Verification items for the finished model (mm, model axes). A direction names the side the tool comes from. Coordinates: 2 decimals unless noted, no trailing zeros. Order: outer loops, then holes, each group sorted by start corner. A loop starts at its lowest first (then second) coordinate and runs counter-clockwise, first axis right, second up. Notation, with made-up numbers: (-17, -5.75) - (11, -5.75) arc R13 cw to (11, 4.25) - close; hole circle Ø5 at (26, 62.5). An arc over 180 degrees is marked (long way). One line per question, with ' | ' between items. Start each with the question number.
from build123d import *

# Parameters (mm, degrees)
RESSALTO_EXTRUS_O1_DEPTH = 2
CORTE_EXTRUS_O1_DEPTH    = 0.1
ESBO_O3_W                = 8
ESBO_O3_H                = 18
ESBO_O3_W_2              = 6.2
ESBO_O3_H_2              = 8.2
RESSALTO_EXTRUS_O2_DEPTH = 1
ESBO_O4_W                = 3.2
ESBO_O4_H                = 1
RESSALTO_EXTRUS_O3_DEPTH = 1.8
ESBO_O5_W                = 3.2
ESBO_O5_H                = 1.4
RESSALTO_EXTRUS_O4_DEPTH = 3
CHANFRO1_SIZE            = 2
CHANFRO1_SIZE2           = 0.388760618
FILETE1_R                = 0.4
ESBO_O6_W                = 3
ESBO_O6_H                = 0.8
RESSALTO_EXTRUS_O5_DEPTH = 1.4
ESBO_O7_W                = 3.5
ESBO_O7_H                = 1.2
CORTE_EXTRUS_O2_DEPTH    = 5


with BuildPart() as part:
    # Esboço1 → Ressalto-extrusão1 (new body)
    with BuildSketch(Plane(origin=(0, 0, 0), x_dir=(1, 0, 0), z_dir=(0, 1, 0))):
        with BuildLine():
            Line((-8.3, -11.4), (8.3, -11.4))
            ThreePointArc((8.3, -11.4), (10.704163056, -10.404163056), (11.7, -8))
            Line((11.7, -8), (11.7, 8))
            ThreePointArc((11.7, 8), (10.704163056, 10.404163056), (8.3, 11.4))
            Line((8.3, 11.4), (-8.3, 11.4))
            ThreePointArc((-8.3, 11.4), (-10.704163056, 10.404163056), (-11.7, 8))
            Line((-11.7, 8), (-11.7, -8))
            ThreePointArc((-11.7, -8), (-10.704163056, -10.404163056), (-8.3, -11.4))
        make_face()
    extrude(amount=RESSALTO_EXTRUS_O1_DEPTH)

    # Esboço2 → Corte-extrusão1 (cut)
    with BuildSketch(Plane(origin=(0, 2, 0), x_dir=(1, 0, 0), z_dir=(0, 1, 0))):
        with BuildLine():
            Line((-8.3, -11), (8.3, -11))
            ThreePointArc((8.3, -11), (10.421320344, -10.121320344), (11.3, -8))
            Line((11.3, -8), (11.3, 8))
            ThreePointArc((11.3, 8), (10.421320344, 10.121320344), (8.3, 11))
            Line((8.3, 11), (-8.3, 11))
            ThreePointArc((-8.3, 11), (-10.421320344, 10.121320344), (-11.3, 8))
            Line((-11.3, 8), (-11.3, -8))
            ThreePointArc((-11.3, -8), (-10.421320344, -10.121320344), (-8.3, -11))
        make_face()
    extrude(amount=-CORTE_EXTRUS_O1_DEPTH, mode=Mode.SUBTRACT)

    # Esboço3 → Ressalto-extrusão2 (add)
    with BuildSketch(Plane(origin=(0, 1.9, 0), x_dir=(1, 0, 0), z_dir=(0, 1, 0))):
        Rectangle(ESBO_O3_W, ESBO_O3_H)
        Rectangle(ESBO_O3_W_2, ESBO_O3_H_2, mode=Mode.SUBTRACT)
    extrude(amount=RESSALTO_EXTRUS_O2_DEPTH)

    # Esboço4 → Ressalto-extrusão3 (add)
    with BuildSketch(Plane(origin=(0, 1.9, 0), x_dir=(1, 0, 0), z_dir=(0, 1, 0))):
        with Locations((5.4, 10.5)):
            Rectangle(ESBO_O4_W, ESBO_O4_H)
    extrude(amount=RESSALTO_EXTRUS_O3_DEPTH)

    # Esboço5 → Ressalto-extrusão4 (add)
    with BuildSketch(Plane(origin=(0, 1.9, 0), x_dir=(1, 0, 0), z_dir=(0, 1, 0))):
        with Locations((-5.4, -10.3)):
            Rectangle(ESBO_O5_W, ESBO_O5_H)
    extrude(amount=RESSALTO_EXTRUS_O4_DEPTH)

    # Chanfro1
    chanfro1_edges = [part.edges().sort_by_distance(p)[0] for p in [
        (-5.4, 4.9, 9.6),
    ]]
    chanfro1_side = [part.faces().sort_by_distance(p)[0] for p in [
        (-5.4, 3.4, 9.6),
    ]]
    chamfer(chanfro1_edges, length=CHANFRO1_SIZE, length2=CHANFRO1_SIZE2, reference=chanfro1_side[0])

    # Filete1
    filete1_edges = [part.edges().sort_by_distance(p)[0] for p in [
        (-5.4, 4.9, 9.988760618),
        (-5.4, 4.9, 11),
    ]]
    fillet(filete1_edges, radius=FILETE1_R)

    # Esboço6 → Ressalto-extrusão5 (add)
    with BuildSketch(Plane(origin=(0, 1.9, 0), x_dir=(1, 0, 0), z_dir=(0, 1, 0))):
        with Locations((8.4, -2.2)):
            Rectangle(ESBO_O6_W, ESBO_O6_H)
    extrude(amount=RESSALTO_EXTRUS_O5_DEPTH)

    # Esboço7 → Corte-extrusão2 (cut)
    with BuildSketch(Plane(origin=(0, 2.9, 0), x_dir=(1, 0, 0), z_dir=(0, 1, 0))):
        with Locations((0, 6.4)):
            Rectangle(ESBO_O7_W, ESBO_O7_H)
        with Locations((0, -6.4)):
            Rectangle(ESBO_O7_W, ESBO_O7_H)
    extrude(amount=-CORTE_EXTRUS_O2_DEPTH, mode=Mode.SUBTRACT)


solid = part.part
Item 1: Set-up check for faces 4 (the flat face through (-1.75, 1, 6)), 5 (the flat face through (0, 2.4, 4.1)), 6 (the flat face through (0, 1, -11.4)): record each of +Z, -Z, +X, -X, +Y, -Y from which the full face is reachable in a straight line by a thin tool's end or side.
Item 2: Thickness scan on probe 1 along X at (y, z) = (2.2, 2); probe 2 along Z at (x, y) = (-1, 0.75); probe 3 along X at (y, z) = (1.3, -6). Record the ranges inside material, lowest first. Write a range as from..to.
Item 3: Section check C-C (x = -1.25). Record the cut outline in (y, z).
Item 4: Gauge pin test, flat ends, axial feed: pin 1 (1.5 mm diameter, centred on x = 2, y = 3, fed in from +Z); pin 2 (0.8 mm diameter, centred on x = 4.5, z = -10.5, fed in from +Y); pin 3 (0.5 mm diameter, centred on y = 3, z = -10.5, fed in from -X). Record the tip position at first contact, or that the pin passes through.
Item 5: Section check D-D (z = 5.25). Record the cut outline in (x, y).
Item 6: Section check B-B (y = 0.7). Record the cut outline in (x, z), then the cut area to 3 significant figures.
Item 7: Mould release check, pull along Z, two halves, no side actions. Record for faces 1 (the flat face through (0, 1, -5.8)), 2 (the cylindrical face through (-10.73, 0.99, 10.38)), 3 (the flat face through (0, 0, 0)): +Z half, -Z half, draft (parallel to the pull), parting line (faces both ways), or undercut.
Item 8: Section check A-A (y = 2.4). Record the cut outline in (x, z), then the cut area to 3 significant figures.
Completed:
1) face 4: +Y, -Y | face 5: +Y | face 6: -Z, +X, -X, +Y, -Y
2) probe 1: x = -4..-3.1, 3.1..4, 6.9..9.9 | probe 2: z = -11.4..-7, -5.8..5.8, 7..11.4 | probe 3: x = -11.7..-1.75, 1.75..11.7
3) outline: (0, -11.4) - (2, -11.4) - (2, -11) - (1.9, -11) - (1.9, -9) - (2.9, -9) - (2.9, -7) - (0, -7) - close; (0, -5.8) - (2.9, -5.8) - (2.9, -4.1) - (1.9, -4.1) - (1.9, 4.1) - (2.9, 4.1) - (2.9, 5.8) - (0, 5.8) - close; (0, 7) - (2.9, 7) - (2.9, 9) - (1.9, 9) - (1.9, 11) - (2, 11) - (2, 11.4) - (0, 11.4) - close
4) pin 1: stops at z = 9 | pin 2: stops at y = 3.7 | pin 3: stops at x = 3.8
5) outline: (-11.7, 0) - (11.7, 0) - (11.7, 2) - (11.3, 2) - (11.3, 1.9) - (4, 1.9) - (4, 2.9) - (-4, 2.9) - (-4, 1.9) - (-11.3, 1.9) - (-11.3, 2) - (-11.7, 2) - close
6) outline: (-11.7, -8) arc R3.4 ccw to (-8.3, -11.4) - (8.3, -11.4) arc R3.4 ccw to (11.7, -8) - (11.7, 8) arc R3.4 ccw to (8.3, 11.4) - (-8.3, 11.4) arc R3.4 ccw to (-11.7, 8) - close; hole (-1.75, -7) - (1.75, -7) - (1.75, -5.8) - (-1.75, -5.8) - close; hole (-1.75, 5.8) - (1.75, 5.8) - (1.75, 7) - (-1.75, 7) - close | area: 515 mm^2
7) face 1: undercut | face 2: +Z half | face 3: draft
8) outline: (-7, 9.6) - (-3.8, 9.6) - (-3.8, 11) - (-7, 11) - close; (-4, -9) - (4, -9) - (4, 9) - (-4, 9) - close; (3.8, -11) - (7, -11) - (7, -10) - (3.8, -10) - close; (6.9, 1.8) - (9.9, 1.8) - (9.9, 2.6) - (6.9, 2.6) - close; hole (-3.1, -4.1) - (3.1, -4.1) - (3.1, 4.1) - (-3.1, 4.1) - close; hole (-1.75, -7) - (1.75, -7) - (1.75, -5.8) - (-1.75, -5.8) - close; hole (-1.75, 5.8) - (1.75, 5.8) - (1.75, 7) - (-1.75, 7) - close | area: 94.8 mm^2
